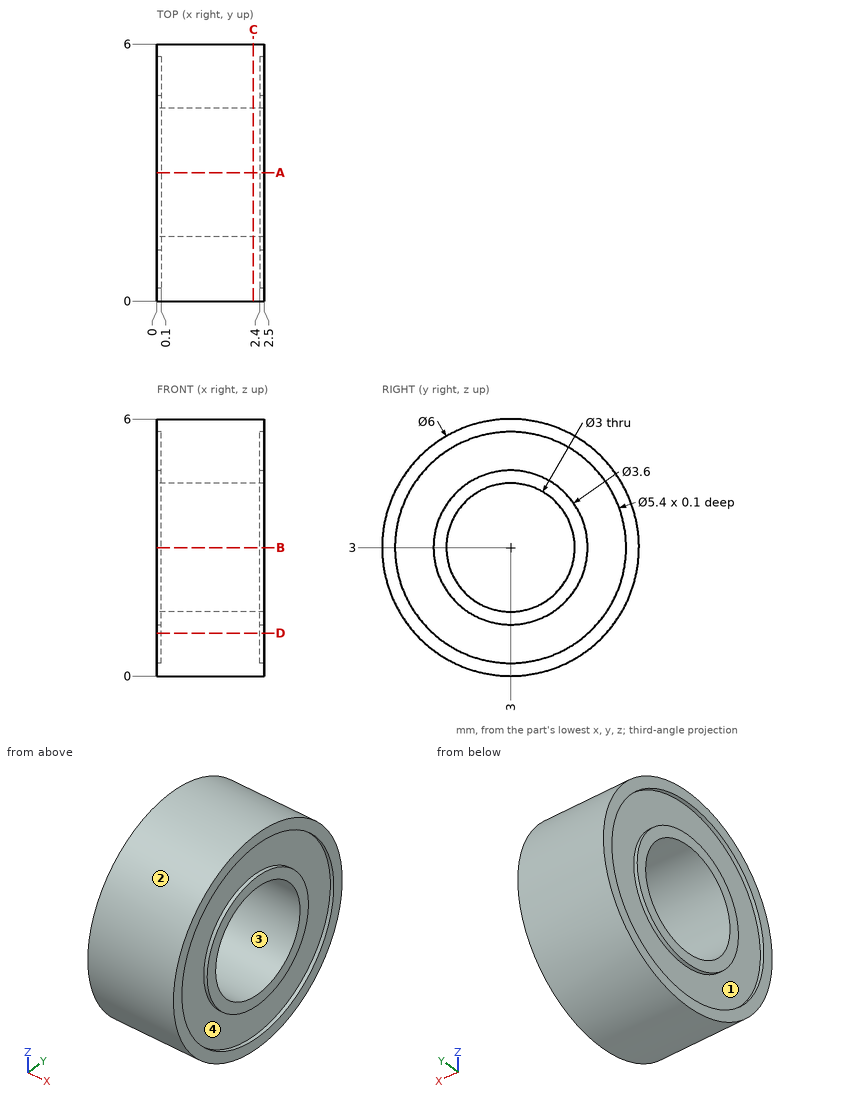
Check sheet for the drawn part. Datum: minimum x, y, z corner. Units: mm. A direction names the side the tool comes from. Round coordinates to 2 decimals unless told otherwise and drop trailing zeros. Write each loop counter-clockwise with the first axis right and the second up, starting at its lowest first coordinate (ties: lowest second). Pieces come first, ordered by that corner, then holes. Notation, with made-up numbers: (86, -10) -> (99, -10) arc R23 cw to (99, 15) -> close; hole circle Ø6 at (-35.75, 78). An arc over 180 degrees is marked (long way). One line per item, written item: value. Start each with the question number.
(1) Cross-section at D-D, the plane z = 1. Record the cut outline in (x, y).
(2) Cross-section at A-A, the plane y = 3. Record the cut outline in (x, z), and give its area (3 significant figures).
(3) Scan lines: line 1 (Y direction, x = 0.05, z = 3); line 2 (Y direction, x = 0.35, z = 1.7); line 3 (X direction, y = 3.4, z = 4.8). Record each from-to range of solid material in increasing order. Write a range as [from, to].
(4) Cross-section at C-C, the plane x = 2.25. Record the cut outline in (y, z), and give its area (3 significant figures).
(5) Draft check along Y on the marked faces 1 and 2. Enter one of: +Y half, -Y half, draft (parallel to the pull), parting line (faces both ways), or undercut.
(6) Access from +Z, -Z, +X, -X, +Y, -Y to the whole of each face (thin tool, end or side, straight path). Record for the marked faces 3 and 4.
Answer:
1. outline: (0, 0.76) -> (2.5, 0.76) -> (2.5, 1.19) -> (2.4, 1.19) -> (2.4, 4.81) -> (2.5, 4.81) -> (2.5, 5.24) -> (0, 5.24) -> (0, 4.81) -> (0.1, 4.81) -> (0.1, 1.19) -> (0, 1.19) -> close
2. outline: (0, 0) -> (2.5, 0) -> (2.5, 0.3) -> (2.4, 0.3) -> (2.4, 1.2) -> (2.5, 1.2) -> (2.5, 1.5) -> (0, 1.5) -> (0, 1.2) -> (0.1, 1.2) -> (0.1, 0.3) -> (0, 0.3) -> close; (0, 4.5) -> (2.5, 4.5) -> (2.5, 4.8) -> (2.4, 4.8) -> (2.4, 5.7) -> (2.5, 5.7) -> (2.5, 6) -> (0, 6) -> (0, 5.7) -> (0.1, 5.7) -> (0.1, 4.8) -> (0, 4.8) -> close
2. area: 7.14 mm²
3. line 1: [0, 0.3], [1.2, 1.5], [4.5, 4.8], [5.7, 6]
3. line 2: [0.3, 2.25], [3.75, 5.7]
3. line 3: [0.1, 2.4]
4. outline: circle Ø6 at (3, 3); hole circle Ø3 at (3, 3)
4. area: 21.2 mm²
5. face 1: undercut
5. face 2: parting line
6. face 3: +X, -X
6. face 4: +X
